from build123d import *

# Parameters (mm, degrees)
SALIENTE_EXTRUIR1_DEPTH = 2
SALIENTE_EXTRUIR2_DEPTH = 4


with BuildPart() as part:
    # Croquis1 → Saliente-Extruir1 (new body)
    with BuildSketch(Plane(origin=(0, 0, 0), x_dir=(1, 0, 0), z_dir=(0, 1, 0))):
        with BuildLine():
            Line((-40.87, -31.3), (40.87, -31.3))
            ThreePointArc((40.87, -31.3), (45.112640687, -29.542640687), (46.87, -25.3))
            Line((46.87, -25.3), (46.87, 25.3))
            ThreePointArc((46.87, 25.3), (45.112640687, 29.542640687), (40.87, 31.3))
            Line((40.87, 31.3), (-40.87, 31.3))
            ThreePointArc((-40.87, 31.3), (-45.112640687, 29.542640687), (-46.87, 25.3))
            Line((-46.87, 25.3), (-46.87, -25.3))
            ThreePointArc((-46.87, -25.3), (-45.112640687, -29.542640687), (-40.87, -31.3))
        make_face()
    extrude(amount=SALIENTE_EXTRUIR1_DEPTH)

    # Croquis2 → Saliente-Extruir2 (add)
    with BuildSketch(Plane(origin=(0, 2, 0), x_dir=(1, 0, 0), z_dir=(0, 1, 0))):
        with BuildLine():
            ThreePointArc((43.87, 25.3), (42.991320344, 27.421320344), (40.87, 28.3))
            Line((40.87, 28.3), (40.87, 29.3))
            ThreePointArc((40.87, 29.3), (43.698427125, 28.128427125), (44.87, 25.3))
            Line((44.87, 25.3), (43.87, 25.3))
        make_face()
        with BuildLine():
            Line((-44.87, 25.3), (-44.37, 25.3))
            ThreePointArc((-44.37, 25.3), (-43.344873734, 27.774873734), (-40.87, 28.8))
            Line((-40.87, 28.8), (-40.87, 29.3))
            ThreePointArc((-40.87, 29.3), (-43.698427125, 28.128427125), (-44.87, 25.3))
        make_face()
        with BuildLine():
            Line((-44.37, 25.3), (-43.87, 25.3))
            ThreePointArc((-43.87, 25.3), (-42.991320344, 27.421320344), (-40.87, 28.3))
            Line((-40.87, 28.3), (-40.87, 28.8))
            ThreePointArc((-40.87, 28.8), (-43.344873734, 27.774873734), (-44.37, 25.3))
        make_face()
        with BuildLine():
            ThreePointArc((-44.87, -25.3), (-43.698427125, -28.128427125), (-40.87, -29.3))
            Line((-40.87, -29.3), (-40.87, -28.3))
            ThreePointArc((-40.87, -28.3), (-42.991320344, -27.421320344), (-43.87, -25.3))
            Line((-43.87, -25.3), (-44.87, -25.3))
        make_face()
        with BuildLine():
            ThreePointArc((43.87, -25.3), (42.991320344, -27.421320344), (40.87, -28.3))
            Line((40.87, -28.3), (40.87, -29.3))
            ThreePointArc((40.87, -29.3), (43.698427125, -28.128427125), (44.87, -25.3))
            Line((44.87, -25.3), (43.87, -25.3))
        make_face()
    extrude(amount=SALIENTE_EXTRUIR2_DEPTH)


solid = part.part
For this review, take the finished solid that the model builds, in its own axes (mm). A direction names the side the tool comes from. Round coordinates to 2 decimals unless told otherwise and drop trailing zeros. Write each loop counter-clockwise with the first axis right and the second up, starting at its lowest first coordinate (ties: lowest second). Pieces come first, ordered by that corner, then holes. Notation, with made-up numbers: (8, 39.25) - (19, 39.25) arc R12 ccw to (19, 55.25) - close; hole circle Ø2 at (49, -11). An arc over 180 degrees is marked (long way). Use a Markdown table: item, result.
Q1. We need section C-C (x = 3). Give the boundary of the cut face in (y, z), plus the area to 3 significant figures.
Derived:
| item | result |
|---|---|
| outline | (0, -31.3) - (2, -31.3) - (2, 31.3) - (0, 31.3) - close |
| area | 125 mm2 |
Q2. We need section D-D (z = -22). Give the boundary of the cut face in (x, y).
Derived:
| item | result |
|---|---|
| outline | (-46.87, 0) - (46.87, 0) - (46.87, 2) - (-46.87, 2) - close |
Q3. The part is to be moulded in two halves that separate along Z. For faces 1 (the flat face through (-1, 1, 31.3)), 2 (the cylindrical face through (-43.01, 3.97, -27.4)), 3 (the flat face through (-43.2, 6, -27.5)), 4 (the cylindrical face through (43.01, 3.97, 27.4)), say which applies: pulls with the +Z half, pulls with the -Z half, needs draft (parallel to the pull), parting line crosses it, or undercut.
Derived:
| item | result |
|---|---|
| face 1 | pulls with the +Z half |
| face 2 | undercut |
| face 3 | needs draft |
| face 4 | undercut |
Q4. Wall thickness on line 1 along Y through (x, z) = (-36.5, -24.5); line 2 along X through (y, z) = (5.6, -25.5) (3 decimals); line 3 along X through (y, z) = (3.75, -27): over which ranges is each line inside the solid? List them lowest first.
Derived:
| item | result |
|---|---|
| line 1 | y = 0 to 2 |
| line 2 | x = -44.865 to -43.863, 43.863 to 44.865 |
| line 3 | x = -44.49 to -43.34, 43.34 to 44.49 |
Q5. Machinability: for faces 5 (the cylindrical face through (-43.729, 3.972, 28.097)), 6 (the cylindrical face through (43.667, 3.972, 28.159)), 7 (the cylindrical face through (43.667, 3.972, -28.159)), which of the approach directions +Z, -Z, +X, -X, +Y, -Y give a long, thin tool a straight path to every point of the face, cutting with its end or side? Answer none if there is none.
Derived:
| item | result |
|---|---|
| face 5 | +Z, -X, +Y |
| face 6 | +Z, +X, +Y |
| face 7 | -Z, +X, +Y |
Q6. Clearance check with flat-ended pins moving along their axes: pin 1 (1.1 mm diameter, centred on y = 4, z = 28.5, fed in from +X); pin 2 (6 mm diameter, centred on x = -16, z = -13.5, fed in from +Y); pin 3 (0.8 mm diameter, centred on y = 3, z = -29, fed in from +X); pin 4 (3 mm diameter, centred on x = 11.5, z = 4.5, fed in from -Y). State where each tip first meets the part, or that it passes through.
Derived:
| item | result |
|---|---|
| pin 1 | stops at x = 43.87 |
| pin 2 | stops at y = 2 |
| pin 3 | stops at x = 43.13 |
| pin 4 | stops at y = 0 |
Q7. We need section A-A (y = 5). Give the boundary of the cut face in (x, z), plus the area to 3 significant figures.
Derived:
| item | result |
|---|---|
| outline | (-44.87, -25.3) arc R4 ccw to (-40.87, -29.3) - (-40.87, -28.3) arc R3 cw to (-43.87, -25.3) - close; (-44.87, 25.3) - (-43.87, 25.3) arc R3 cw to (-40.87, 28.3) - (-40.87, 29.3) arc R4 ccw to start; (40.87, -29.3) arc R4 ccw to (44.87, -25.3) - (43.87, -25.3) arc R3 cw to (40.87, -28.3) - close; (40.87, 28.3) arc R3 cw to (43.87, 25.3) - (44.87, 25.3) arc R4 ccw to (40.87, 29.3) - close |
| area | 22.0 mm2 |
Q8. We need section B-B (z = 27). Give the boundary of the cut face in (x, y), plus the area to 3 significant figures.
Derived:
| item | result |
|---|---|
| outline | (-46.62, 0) - (46.62, 0) - (46.62, 2) - (44.49, 2) - (44.49, 6) - (43.34, 6) - (43.34, 2) - (-43.34, 2) - (-43.34, 6) - (-44.49, 6) - (-44.49, 2) - (-46.62, 2) - close |
| area | 196 mm2 |
